Answer from the drawing. Dimensions are ordinates in mm from the lowest x, y and z of the part. Give positions to 0.01 mm unless a question says otherwise; leave off trailing zeros. Order: outer loops, then holes, each group sorted by start corner. A loop starts at its lowest first (then second) coordinate and runs counter-clockwise, first axis right, second up. Notation, with made-up numbers: M 80.25,-2 L 117.25,-2 A33 cw 117.25,26 Z; hole C 6,-7.5 d2. An arc over 180 degrees is marked long. One line per item, written item: value.
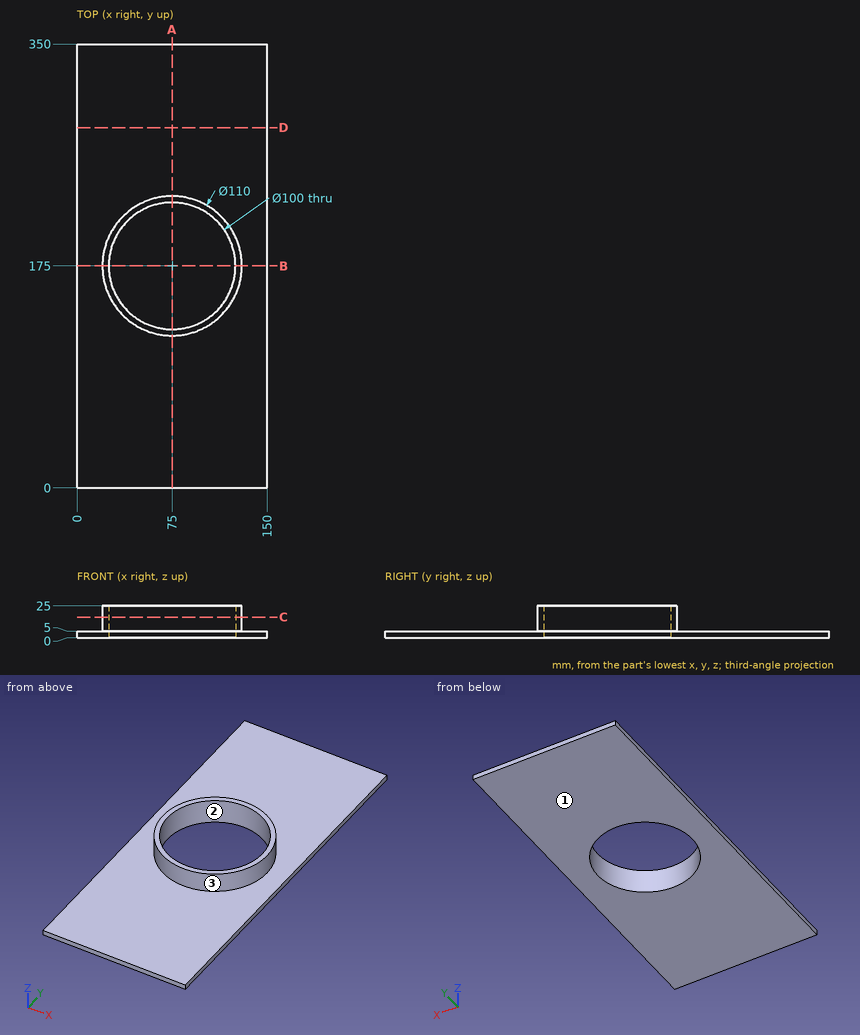
(1) Section B-B, the plane y = 175 is taken. Give the vertices of the cut face in (x, z), then the cut area to 3 significant figures.
Findings:
outline: M 0,0 L 25,0 L 25,25 L 20,25 L 20,5 L 0,5 Z; M 125,0 L 150,0 L 150,5 L 130,5 L 130,25 L 125,25 Z
area: 450 mm^2
(2) Section D-D, the plane y = 284 is taken. Give the vertices of the cut face in (x, z).
Findings:
outline: M 0,0 L 150,0 L 150,5 L 0,5 Z
(3) Determine the mould class of the marked faces 1, 2 and 3 for opening direction X: pulls with the +X half, pulls with the -X half, needs draft (parallel to the pull), parting line crosses it, or undercut.
Findings:
face 1: needs draft
face 2: undercut
face 3: parting line crosses it
(4) Find the intervals of material crossed by probe 1 along Y at (x, z) = (75, 8.5); probe 2 along Z at (x, y) = (8.5, 271); probe 3 along Y at (x, z) = (79, 23.25), in increasing order. Write a range as from..to.
Findings:
probe 1: y = 120..125, 225..230
probe 2: z = 0..5
probe 3: y = 120.15..125.16, 224.84..229.85
(5) Section A-A, the plane x = 75 is taken. Give the vertices of the cut face in (y, z).
Findings:
outline: M 0,0 L 125,0 L 125,25 L 120,25 L 120,5 L 0,5 Z; M 225,0 L 350,0 L 350,5 L 230,5 L 230,25 L 225,25 Z
(6) Section C-C, the plane z = 16 is taken. Give the vertices of the cut face in (x, y).
Findings:
outline: C 75,175 d110; hole C 75,175 d100
(7) Given P1, Ø2, axis at x = 97, z = 19.5, coming from the -Y side, flat-ended and moving along its own axis, determine where the tip first touches the part or whether it passes through.
Findings:
P1: stops at y = 124.17
